from build123d import *

# Parameters (mm, degrees)
F2_W     = 6.35
F2_H     = 6.35
F3_DEPTH = 63.501
F4_R     = 6.35
F5_DEPTH = 31.75


with BuildPart() as f1:
    # F0 (on Front) → F1 (revolve)
    with BuildSketch(Plane.XZ):
        Polygon((0, 20.32), (0, 12.7), (63.5, 12.7), (63.5, 69.85), (57.15, 69.85), (57.15, 20.32), align=None)
    revolve(axis=Axis((31.75, 0, 0), (1, 0, 0)))

    # F2 (on Right) → F3 (cut, through all)
    with BuildSketch(Plane.YZ):
        with Locations((0, 12.7)):
            Rectangle(F2_W, F2_H)
    extrude(amount=F3_DEPTH, mode=Mode.SUBTRACT)

    # F4 (on face) → F5 (join)
    with BuildSketch(Plane.YZ.offset(63.5)):
        with Locations((0, 50.8)):
            Circle(F4_R)
        with Locations((-50.8, 0)):
            Circle(F4_R)
        with Locations((0, -50.8)):
            Circle(F4_R)
        with Locations((50.8, 0)):
            Circle(F4_R)
    extrude(amount=F5_DEPTH)


solid = f1.part
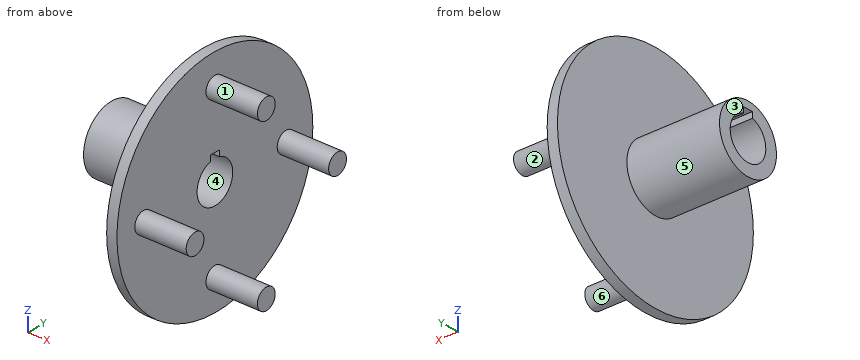
Could you check a few things on this model? Use its own coordinates, in mm. Face numbers are marked on the shaded views. A direction names the side the tool comes from. Give positions to 0.01 mm unless a question says otherwise; leave off trailing zeros. Loops run counter-clockwise (first coordinate to the right, second up) from the corner with the lowest first, then second, coordinate; pieces in that order, holes last. Notation, with made-up numbers: (14, -6.5) -> (53, -6.5) arc R9 cw to (53, 1.5) -> close; hole circle Ø4 at (13.5, -11.5). An arc over 180 degrees is marked (long way). Answer as CSV lines item,"result". Start each with the question number.
(1) We'd pull the mould along Z, two halves only. Please class the marked faces 1, 2 and 3: released by +Z, released by -Z, zero draft, split by the parting line, or undercut.
(2) I'm going to push flat-ended pins straight in: pin 1 Ø12 at (x, y) = (83.5, 0) entering from -Z; pin 2 Ø10 at (y, z) = (49, 14) entering from +X; pin 3 Ø3 at (x, z) = (42.5, 14) entering from -Y. Where does each tip first touch, or does it pass through?
(3) If we section it at C-C on x = 33: Write out the boundary of the cut face in (y, z) (3 decimals).
(4) If we section it at D-D on z = 50.8: Write out the boundary of the cut face in (x, y).
(5) If we section it at B-B on y = 0: Write out the boundary of the cut face in (x, z) (3 decimals), then the cut area to 3 significant figures.
(6) I need wall thicknesses on probe 1 along Z at (x, y) = (40, 0) (3 decimals); probe 2 along Y at (x, z) = (20, 0); probe 3 along X at (y, z) = (40, -48). Which ranges of each line are inside material? Lowest first, please.
(7) Which directions (+Z, -Z, +X, -X, +Y, -Y) give clear straight access to the entire face, cutting with the end or side of a thin tool? Please do the marked faces 4, 5 and 6.
(8) If we section it at A-A on z = 0: Write out the boundary of the cut face in (x, y).
Computed:
1,face 1,"undercut"
1,face 2,"split by the parting line"
1,face 3,"zero draft"
2,pin 1,"stops at z = -57.15"
2,pin 2,"stops at x = 63.5"
2,pin 3,"stops at y = -16.02"
3,outline,"circle Ø40.64 at (0, 0); hole (-3.175, 12.297) arc R12.7 ccw (long way) to (3.175, 12.297) -> (3.175, 15.875) -> (-3.175, 15.875) -> close"
4,outline,"(57.15, -47.94) -> (63.5, -47.94) -> (63.5, -6.35) -> (95.25, -6.35) -> (95.25, 6.35) -> (63.5, 6.35) -> (63.5, 47.94) -> (57.15, 47.94) -> close"
5,outline,"(0, -20.32) -> (57.15, -20.32) -> (57.15, -69.85) -> (63.5, -69.85) -> (63.5, -57.15) -> (95.25, -57.15) -> (95.25, -44.45) -> (63.5, -44.45) -> (63.5, -12.7) -> (0, -12.7) -> close; (0, 15.875) -> (63.5, 15.875) -> (63.5, 44.45) -> (95.25, 44.45) -> (95.25, 57.15) -> (63.5, 57.15) -> (63.5, 69.85) -> (57.15, 69.85) -> (57.15, 20.32) -> (0, 20.32) -> close"
5,area,"2,200 mm2"
6,probe 1,"z = -20.32 to -12.7, 15.875 to 20.32"
6,probe 2,"y = -20.32 to -12.7, 12.7 to 20.32"
6,probe 3,"x = 57.15 to 63.5"
7,face 4,"+X, -X"
7,face 5,"-X"
7,face 6,"+X"
8,outline,"(0, -20.32) -> (57.15, -20.32) -> (57.15, -69.85) -> (63.5, -69.85) -> (63.5, -57.15) -> (95.25, -57.15) -> (95.25, -44.45) -> (63.5, -44.45) -> (63.5, -12.7) -> (0, -12.7) -> close; (0, 12.7) -> (63.5, 12.7) -> (63.5, 44.45) -> (95.25, 44.45) -> (95.25, 57.15) -> (63.5, 57.15) -> (63.5, 69.85) -> (57.15, 69.85) -> (57.15, 20.32) -> (0, 20.32) -> close"
